Can you work these out from the model? Positions are in its coordinate system, mm. A direction names the side the tool comes from. Give positions to 0.01 mm unless a question says otherwise; leave off trailing zeros. Write each loop counter-clockwise with the first axis right and the second up, starting at its lowest first coordinate (ties: lowest second). Pieces come first, ordered by that corner, then holes. Notation, with made-up numbers: M 22,62.25 L 73,62.25 A31 cw 73,92.25 Z; hole C 46,-16 d1. An arc over 180 degrees is marked long. Write each question's results on one line, items separated by ' | '.
from build123d import *

# Parameters (mm, degrees)
F0_W     = 50
F0_H     = 50
F1_DEPTH = 50
F2_R     = 10
F3_DEPTH = 15
F4_T     = -2.5


with BuildPart() as f1:
    # F0 (on Top) → F1 (new body)
    with BuildSketch(Plane.XY):
        Rectangle(F0_W, F0_H)
    extrude(amount=F1_DEPTH)

    # F2
    f2_edges = [f1.edges().sort_by_distance(p)[0] for p in [
        (-25, -25, 25),
        (-25, 25, 25),
        (25, 25, 25),
        (25, -25, 25),
    ]]
    fillet(f2_edges, radius=F2_R)

    # F1_face (on face) → F3 (join)
    with BuildSketch(Plane(origin=(0, 0, 0), x_dir=(1, 0, 0), z_dir=(0, 0, -1))):
        with BuildLine():
            Line((-25, 15), (-25, -15))
            ThreePointArc((-25, -15), (-22.071068, -22.071068), (-15, -25))
            Line((-15, -25), (15, -25))
            ThreePointArc((15, -25), (22.071068, -22.071068), (25, -15))
            Line((25, -15), (25, 15))
            ThreePointArc((25, 15), (22.071068, 22.071068), (15, 25))
            Line((15, 25), (-15, 25))
            ThreePointArc((-15, 25), (-22.071068, 22.071068), (-25, 15))
        make_face()
    extrude(amount=F3_DEPTH)

    # F4
    f4_openings = [f1.faces().sort_by_distance(p)[0] for p in [
        (0, 0, 50),
    ]]
    offset(amount=F4_T, openings=f4_openings)


solid = f1.part
Item 1: I want a section at B-B, the plane y = 7. Please give me the cut outline in (x, z), and give its area (4 significant figures).
Geometry says:
outline: M -25,-15 L 25,-15 L 25,50 L 22.5,50 L 22.5,-12.5 L -22.5,-12.5 L -22.5,50 L -25,50 Z | area: 437.5 mm2
Item 2: I want a section at D-D, the plane x = -17.5. Please give me the cut outline in (y, z).
Geometry says:
outline: M -24.68,-15 L 24.68,-15 L 24.68,50 L 22.07,50 L 22.07,-12.5 L -22.07,-12.5 L -22.07,50 L -24.68,50 Z
Item 3: If I drill on line 1 (Y direction, x = -2.5, z = 9.5); line 2 (X direction, y = 15.5, z = 36.5); line 3 (Z direction, x = -1, y = -19.5), over which ranges is the centre line in solid material (lowest first)? Write a range as from..to.
Geometry says:
line 1: y = -25..-22.5, 22.5..25 | line 2: x = -24.99..-22.48, 22.48..24.99 | line 3: z = -15..-12.5
Item 4: I want a section at A-A, the plane z = -8. Please give me the cut outline in (x, y).
Geometry says:
outline: M -25,-15 A10 ccw -15,-25 L 15,-25 A10 ccw 25,-15 L 25,15 A10 ccw 15,25 L -15,25 A10 ccw -25,15 Z; hole M -22.5,-15 A7.5 ccw -15,-22.5 L 15,-22.5 A7.5 ccw 22.5,-15 L 22.5,15 A7.5 ccw 15,22.5 L -15,22.5 A7.5 ccw -22.5,15 Z
Item 5: Thinking about a two-plate mould opening in Y: for faces 3 (the face through (-22.5, 0, 19)), 4 (the face through (25, 0, 18)), 5 (the face through (0, 25, 18)), 6 (the face through (22.5, 0, 19)), which applies, +Y half, -Y half, draft (parallel to the pull), parting line (faces both ways), or undercut?
Geometry says:
face 3: undercut | face 4: draft | face 5: +Y half | face 6: undercut
Item 6: I'm going to push flat-ended pins straight in: pin 1 (6 mm diameter, centred on y = -20, z = 28.5, fed in from -X); pin 2 (2 mm diameter, centred on x = 3, y = -18.5, fed in from +Z); pin 3 (2 mm diameter, centred on y = -16.5, z = 36.5, fed in from +X). Where does each tip first touch, or does it pass through?
Geometry says:
pin 1: stops at x = -24.8 | pin 2: stops at z = -12.5 | pin 3: stops at x = 24.99
Item 7: For faces 1 (the face through (-25, 0, 18)), 2 (the face through (0, 0, -12.5)), which set-ups out of +Z, -Z, +X, -X, +Y, -Y let a thin tool reach every point of the face, with its end or its side?
Geometry says:
face 1: +Z, -Z, -X, +Y, -Y | face 2: +Z
